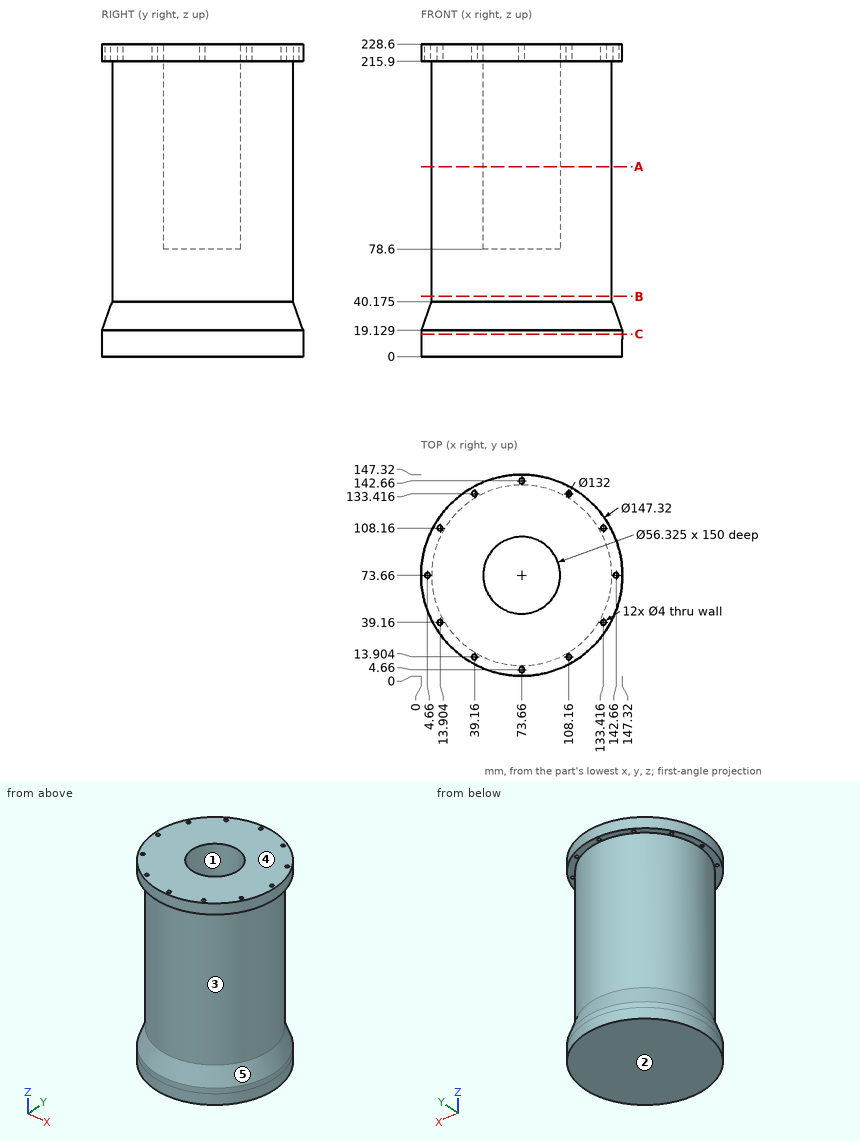
Source: three-view drawing plus pictorial views. Frame: mm from the lowest corner of the part. A direction names the side the tool comes from. Round coordinates to 2 decimals unless told otherwise and drop trailing zeros. Write each loop counter-clockwise with the first axis right and the second up, starting at its lowest first coordinate (ties: lowest second). Pieces come first, ordered by that corner, then holes. Notation, with made-up numbers: M -22,15 L 14,15 A20 cw 14,52 Z; hole C -16.75,62.5 d7. An arc over 180 degrees is marked long. One line per item, written item: value. Start each with the question number.
Item 1: Pin query (flat end, axial travel): pin 1 (12 mm diameter, centred on x = 52.5, y = 77, fed in from +Z); pin 2 (5 mm diameter, centred on y = 112, z = 95, fed in from +X); pin 3 (12 mm diameter, centred on x = 53, z = 190, fed in from +Y). Return the tip coordinate at first contact, or that it passes through.
Item 2: Section query C-C (z = 16.5). Return the cut outline in (x, y), plus the area to 3 significant figures.
Item 3: Ray query, L1, parallel to Y at x = 73, z = 221 (1 decimal); L2, parallel to Y at x = 39.16, z = 220.75 (1 decimal); L3, parallel to Z at x = 78, y = 67.5. Return the intervals inside material, ascending. Write a range as from..to.
Item 4: Mould query, pull axis Y, two halves, no side actions, for the marked faces 1, 2 and 3. Classes: pulls with the +Y half, pulls with the -Y half, needs draft (parallel to the pull), parting line crosses it, or undercut.
Item 5: Section query A-A (z = 139). Return the cut outline in (x, y) (1 decimal), plus the area to 3 significant figures.
Item 6: Section query B-B (z = 44). Return the cut outline in (x, y), plus the area to 3 significant figures.
Item 7: Set-up query: the marked faces 4 and 5. Return all of +Z, -Z, +X, -X, +Y, -Y with unobstructed straight access to the full face (end or side cutting, diameter ignored); none if empty.
Result set:
1. pin 1: stops at z = 78.6
1. pin 2: stops at x = 129.08
1. pin 3: stops at y = 138.01
2. outline: C 73.66,73.66 d147.32
2. area: 17,000 mm²
3. L1: y = 0..2.8, 6.5..45.5, 101.8..140.8, 144.5..147.3
3. L2: y = 8.6..11.9, 15.9..131.4, 135.4..138.7
3. L3: z = 0..78.6
4. face 1: undercut
4. face 2: needs draft
4. face 3: parting line crosses it
5. outline: C 73.7,73.7 d132; hole C 73.7,73.7 d56.3
5. area: 11,200 mm²
6. outline: C 73.66,73.66 d132
6. area: 13,700 mm²
7. face 4: +Z, +X, -X, +Y, -Y
7. face 5: none
